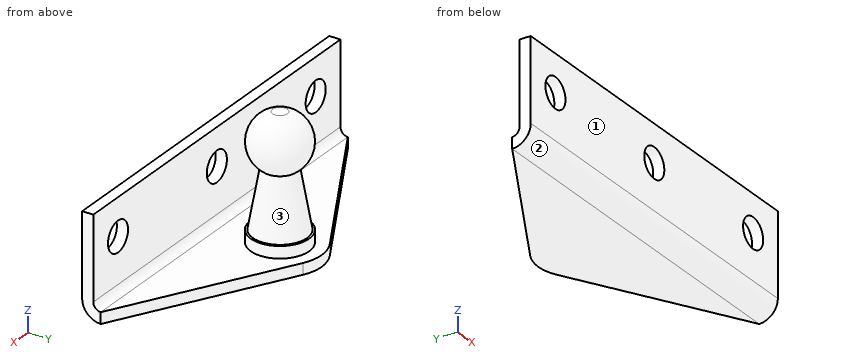
```python
from build123d import *

# Parameters (mm, degrees)
EXTRUDE1_DEPTH     = 1.905
SKETCH4_W          = 63.5
SKETCH4_H          = 17.272
EXTRUDE2_DEPTH     = 1.905
FILLET1_R          = 1.27
FILLET2_R          = 3.175
SKETCH5_R          = 2.5781
CUT_EXTRUDE1_DEPTH = 42.217712552


with BuildPart() as part:
    # Sketch1 → Extrude1 (new body)
    with BuildSketch(Plane.XY):
        with BuildLine():
            Line((-31.75, -12.7), (31.75, -12.7))
            Line((31.75, -12.7), (31.75, -9.525))
            Line((31.75, -9.525), (3.457575677, 6.214958925))
            ThreePointArc((3.457575677, 6.214958925), (0, 7.112), (-3.457575677, 6.214958925))
            Line((-3.457575677, 6.214958925), (-31.75, -9.525))
            Line((-31.75, -9.525), (-31.75, -12.7))
        make_face()
    extrude(amount=EXTRUDE1_DEPTH)

    # Sketch4 → Extrude2 (add)
    with BuildSketch(Plane.XZ.offset(12.7)):
        with Locations((0, 8.636)):
            Rectangle(SKETCH4_W, SKETCH4_H)
    extrude(amount=-EXTRUDE2_DEPTH)

    # Fillet1
    fillet1_edges = [part.edges().sort_by_distance(p)[0] for p in [
        (0, -10.795, 1.905),
    ]]
    fillet(fillet1_edges, radius=FILLET1_R)

    # Fillet2
    fillet2_edges = [part.edges().sort_by_distance(p)[0] for p in [
        (0, -12.7, 0),
    ]]
    fillet(fillet2_edges, radius=FILLET2_R)

    # Sketch5 → Cut-Extrude1 (cut, through all)
    with BuildSketch(Plane.XZ.offset(12.7)):
        with Locations((-25.4, 10.922)):
            Circle(SKETCH5_R)
        with Locations((25.4, 10.922)):
            Circle(SKETCH5_R)
        with Locations((0, 10.922)):
            Circle(SKETCH5_R)
    extrude(amount=-CUT_EXTRUDE1_DEPTH, mode=Mode.SUBTRACT)

    # Sketch3 → Revolve1 (revolve)
    with BuildSketch(Plane.XZ):
        with BuildLine():
            Line((0, 1.905), (0, 22.987))
            Line((0, 22.987), (1.27, 22.987))
            ThreePointArc((1.27, 22.987), (4.92353173, 19.022090442), (2.852216719, 14.044294139))
            Line((2.852216719, 14.044294139), (4.640481928, 3.937))
            Line((4.640481928, 3.937), (5, 3.937))
            Line((5, 3.937), (5, 1.905))
            Line((5, 1.905), (0, 1.905))
        make_face()
    revolve(axis=Axis((0, 0, 1.905), (0, 0, -1)))


solid = part.part
```
The listing builds one solid part. Answer for the finished solid, in the listing's coordinates (mm). Face numbers are marked on the shaded views. Round coordinates to 2 decimals unless told otherwise and drop trailing zeros. Loops run counter-clockwise (first coordinate to the right, second up) from the corner with the lowest first, then second, coordinate; pieces in that order, holes last.
Q1. Section D-D, the plane x = 15 is taken. Determine the outline of the cut face in (y, z) (3 decimals), then the cut area to 3 significant figures.
Q2. Find the intervals of material crossed by line 1 (Z direction, x = -24, y = -6.5) (3 decimals); line 2 (Y direction, x = 13, z = 12.25) (3 decimals); line 3 (Y direction, x = 2, z = 3), in increasing order.
Q3. Section C-C, the plane y = 0 is taken. Determine the outline of the cut face in (x, z) (3 decimals), then the cut area to 3 significant figures.
Q4. Section B-B, the plane z = 12 is taken. Determine the outline of the cut face in (x, y) (3 decimals), then the cut area to 3 significant figures.
Q5. For a pull along Z with two mould halves and no side action, classify the marked faces 1, 2 and 3 as released by +Z, released by -Z, zero draft, split by the parting line, or undercut.
Q6. Section A-A, the plane x = -25.4 is taken. Determine the outline of the cut face in (y, z) (3 decimals), then the cut area to 3 significant figures.
Q7. Given pin 1 Ø2 at (x, y) = (-13, -12) entering from +Z; pin 2 Ø1 at (x, z) = (-4.5, 8.5) entering from +Y (3 decimals); pin 3 Ø11.5 at (x, z) = (10, 8.5) entering from +Y, each flat-ended and moving along its own axis, determine where each tip first touches the part or whether it passes through.
Completed:
1. outline: (-12.7, 3.175) arc R3.175 ccw to (-9.525, 0) - (-0.206, 0) - (-0.206, 1.905) - (-9.525, 1.905) arc R1.27 cw to (-10.795, 3.175) - (-10.795, 17.272) - (-12.7, 17.272) - close
1. area: 51.3 mm2
2. line 1: z = 0 to 1.905
2. line 2: y = -12.7 to -10.795
2. line 3: y = -12.7 to -10.78, -4.58 to 4.58
3. outline: (-14.629, 0) - (14.629, 0) - (14.629, 1.905) - (5, 1.905) - (5, 3.937) - (4.64, 3.937) - (2.852, 14.044) arc R5 ccw to (1.27, 22.987) - (-1.27, 22.987) arc R5 ccw to (-2.852, 14.044) - (-4.64, 3.937) - (-5, 3.937) - (-5, 1.905) - (-14.629, 1.905) - close
3. area: 227 mm2
4. outline: (-31.75, -12.7) - (-27.742, -12.7) - (-27.742, -10.795) - (-31.75, -10.795) - close; (-23.058, -12.7) - (-2.342, -12.7) - (-2.342, -10.795) - (-23.058, -10.795) - close; circle Ø6.428 at (0, 0); (2.342, -12.7) - (23.058, -12.7) - (23.058, -10.795) - (2.342, -10.795) - close; (27.742, -12.7) - (31.75, -12.7) - (31.75, -10.795) - (27.742, -10.795) - close
4. area: 127 mm2
5. face 1: zero draft
5. face 2: released by -Z
5. face 3: undercut
6. outline: (-12.7, 3.175) arc R3.175 ccw to (-9.525, 0) - (-5.992, 0) - (-5.992, 1.905) - (-9.525, 1.905) arc R1.27 cw to (-10.795, 3.175) - (-10.795, 8.344) - (-12.7, 8.344) - close; (-12.7, 13.5) - (-10.795, 13.5) - (-10.795, 17.272) - (-12.7, 17.272) - close
6. area: 30.4 mm2
7. pin 1: stops at z = 17.27
7. pin 2: stops at y = -10.795
7. pin 3: stops at y = -10.72
